```python
from build123d import *

# Parameters (mm, degrees)
F0_W     = 450
F0_H     = 180
F1_DEPTH = 10
F2_W     = 420
F2_H     = 160
F2_W_2   = 400
F2_H_2   = 140
F3_DEPTH = 70
F5_D     = 16.5


with BuildPart() as f1:
    # F0 (on Top) → F1 (new body)
    with BuildSketch(Plane.XY):
        Rectangle(F0_W, F0_H)
    extrude(amount=F1_DEPTH)

    # F2 (on face) → F3 (join)
    with BuildSketch(Plane(origin=(0, 0, 0), x_dir=(1, 0, 0), z_dir=(0, 0, -1))):
        Rectangle(F2_W, F2_H)
        Rectangle(F2_W_2, F2_H_2, mode=Mode.SUBTRACT)
    extrude(amount=F3_DEPTH)

    # F5 (through all)
    with Locations(Plane.XY.offset(10)):
        with Locations((-185, -55), (-155, -55)):
            Hole(F5_D / 2)


solid = f1.part
```
CAD build for the part. Positions are in the model's coordinates, mm. A direction names the side the tool comes from. Round coordinates to 2 decimals unless told otherwise and drop trailing zeros. Order: outer loops, then holes, each group sorted by start corner. A loop starts at its lowest first (then second) coordinate and runs counter-clockwise, first axis right, second up. Notation, with made-up numbers: (42, 51.5) - (86, 51.5) arc R25 ccw to (86, 77.5) - close; hole circle Ø7 at (42, -18). An arc over 180 degrees is marked (long way). Use CSV: the item, a comma, the result in double quotes. Start each with the question number.
1) Saw through at C-C (z = -26). List the corners of the cut face in (x, y), and give its area (3 significant figures).
2) Pin check, flat tips, straight feed: pin 1 Ø10 at (x, z) = (72, -50) entering from +Y; pin 2 Ø3 at (y, z) = (-58.5, -59.5) entering from +X; pin 3 Ø5 at (x, z) = (35.5, -1.5) entering from -Y; pin 4 Ø8 at (y, z) = (33.5, -37) entering from -X. Stop position of each tip, or through.
3) Saw through at B-B (y = -55). List the corners of the cut face in (x, z).
4) Saw through at D-D (x = 42). List the corners of the cut face in (y, z), and give its area (3 significant figures).
5) Wall check: L1, parallel to Y at x = 69.5, z = -20.5; L2, parallel to X at y = 31, z = -12.5; L3, parallel to Y at x = -185, z = 3. Give the ranges that are in metal, low to high. Write a range as [from, to].
6) Two-plate mould, pull along Y, no slides. Class faces 1 (the flat face through (-210, 1, -35)), 2 (the flat face through (-3, -80, -35)), 3 (the flat face through (-200, 1, -35)), 4 (the flat face through (-3, 90, 5)): pulls with the +Y half, pulls with the -Y half, needs draft (parallel to the pull), parting line crosses it, or undercut.
7) Tool access for faces 5 (the flat face through (-3, 80, -35)), 6 (the flat face through (210, 1, -35)), 7 (the flat face through (-3, 1, 0)), 8 (the flat face through (-225, -1, 5)), 9 (the flat face through (-17, 71, -70)): list every direction of +Z, -Z, +X, -X, +Y, -Y with a clear straight run to the whole face (end or side of a thin tool).
8) Saw through at A-A (x = -185). List the corners of the cut face in (y, z), and give its area (4 significant figures).
Values follow:
1,outline,"(-210, -80) - (210, -80) - (210, 80) - (-210, 80) - close; hole (-200, -70) - (200, -70) - (200, 70) - (-200, 70) - close"
1,area,"11,200 mm2"
2,pin 1,"stops at y = 80"
2,pin 2,"stops at x = 210"
2,pin 3,"stops at y = -90"
2,pin 4,"stops at x = -210"
3,outline,"(-225, 0) - (-210, 0) - (-210, -70) - (-200, -70) - (-200, 0) - (-193.25, 0) - (-193.25, 10) - (-225, 10) - close; (-176.75, 0) - (-163.25, 0) - (-163.25, 10) - (-176.75, 10) - close; (-146.75, 0) - (200, 0) - (200, -70) - (210, -70) - (210, 0) - (225, 0) - (225, 10) - (-146.75, 10) - close"
4,outline,"(-90, 0) - (-80, 0) - (-80, -70) - (-70, -70) - (-70, 0) - (70, 0) - (70, -70) - (80, -70) - (80, 0) - (90, 0) - (90, 10) - (-90, 10) - close"
4,area,"3,200 mm2"
5,L1,"y = [-80, -70], [70, 80]"
5,L2,"x = [-210, -200], [200, 210]"
5,L3,"y = [-90, -63.25], [-46.75, 90]"
6,face 1,"needs draft"
6,face 2,"pulls with the -Y half"
6,face 3,"undercut"
6,face 4,"pulls with the +Y half"
7,face 5,"-Z, +X, -X, +Y"
7,face 6,"-Z, +X, +Y, -Y"
7,face 7,"-Z"
7,face 8,"+Z, -Z, -X, +Y, -Y"
7,face 9,"-Z, +X, -X, +Y, -Y"
8,outline,"(-90, 0) - (-80, 0) - (-80, -70) - (-70, -70) - (-70, 0) - (-63.25, 0) - (-63.25, 10) - (-90, 10) - close; (-46.75, 0) - (70, 0) - (70, -70) - (80, -70) - (80, 0) - (90, 0) - (90, 10) - (-46.75, 10) - close"
8,area,"3,035 mm2"
